Check sheet for the modelled part. Datum: model origin and axes. Units: mm. Face numbers are marked on the shaded views. A direction names the side the tool comes from. Coordinates: 2 decimals unless noted, no trailing zeros. Loops run counter-clockwise (first coordinate to the right, second up) from the corner with the lowest first, then second, coordinate; pieces in that order, holes last. Notation, with made-up numbers: M -38,44.5 L -29,44.5 A8 cw -29,52.5 Z; hole C 76.25,53 d6. An arc over 180 degrees is marked long. Return JSON: item names as keys, results as strings.
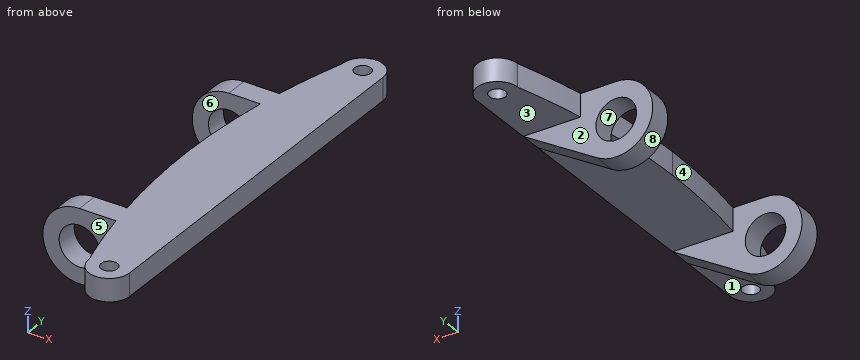
from build123d import *

# Parameters (mm, degrees)
CROQUIS3_R              = 1
SALIENTE_EXTRUIR1_DEPTH = 2.8
SALIENTE_EXTRUIR2_START = 12.5
CROQUIS4_R              = 2.5
SALIENTE_EXTRUIR2_DEPTH = 2.8
SALIENTE_EXTRUIR3_START = -15.3
CROQUIS4_2_R            = 2.5
SALIENTE_EXTRUIR3_DEPTH = 2.8


with BuildPart() as part:
    # Croquis3 → Saliente-Extruir1 (new body)
    with BuildSketch(Plane.XY):
        with BuildLine():
            Line((4.846627727, 23.897818016), (4.846627727, -23.274751548))
            ThreePointArc((4.846627727, -23.274751548), (2.346627727, -25.774751548), (-0.153372273, -23.274751548))
            ThreePointArc((-0.153372273, -23.274751548), (-2.736363907, -11.605217887), (-3.653372273, 0.311533234))
            ThreePointArc((-3.653372273, 0.311533234), (-2.736363907, 12.228284355), (-0.153372273, 23.897818016))
            ThreePointArc((-0.153372273, 23.897818016), (2.346627727, 26.397818016), (4.846627727, 23.897818016))
        make_face()
        with Locations((2.346627727, 23.897818016)):
            Circle(CROQUIS3_R, mode=Mode.SUBTRACT)
        with Locations(Location((2.346627727, -23.274751548, 0), (0, 0, 180))):
            Circle(CROQUIS3_R, mode=Mode.SUBTRACT)
    extrude(amount=SALIENTE_EXTRUIR1_DEPTH)

    # Croquis4 → Saliente-Extruir2 (add)
    with BuildSketch(Plane(origin=(0, 0, 0), x_dir=(1, 0, 0), z_dir=(0, 1, 0)).offset(SALIENTE_EXTRUIR2_START)):
        with BuildLine():
            Line((4.846627727, 0), (-4.267297244, 5.544479263))
            ThreePointArc((-4.267297244, 5.544479263), (-10.939117757, 2.914463527), (-6.606095909, -2.8))
            Line((-6.606095909, -2.8), (-3.653372273, -2.8))
            Line((-3.653372273, -2.8), (4.846627727, -2.8))
            Line((4.846627727, -2.8), (4.846627727, 0))
        make_face()
        with Locations(Location((-6.606095909, 1.7, 0), (0, 0, 270))):
            Circle(CROQUIS4_R, mode=Mode.SUBTRACT)
    extrude(amount=SALIENTE_EXTRUIR2_DEPTH)

    # Croquis4_2 → Saliente-Extruir3 (add)
    with BuildSketch(Plane(origin=(0, 0, 0), x_dir=(1, 0, 0), z_dir=(0, 1, 0)).offset(SALIENTE_EXTRUIR3_START)):
        with BuildLine():
            Line((4.846627727, 0), (-4.267297244, 5.544479263))
            ThreePointArc((-4.267297244, 5.544479263), (-10.939117757, 2.914463527), (-6.606095909, -2.8))
            Line((-6.606095909, -2.8), (-3.653372273, -2.8))
            Line((-3.653372273, -2.8), (4.846627727, -2.8))
            Line((4.846627727, -2.8), (4.846627727, 0))
        make_face()
        with Locations(Location((-6.606095909, 1.7, 0), (0, 0, 270))):
            Circle(CROQUIS4_2_R, mode=Mode.SUBTRACT)
    extrude(amount=SALIENTE_EXTRUIR3_DEPTH)


solid = part.part
1) Go/stop test with flat-tipped pins: pin 1 Ø1.8 at (x, y) = (2.35, 23.9) entering from +Z; pin 2 Ø8 at (x, y) = (-6, -3) entering from -Z; pin 3 Ø5 at (x, z) = (1.5, -3) entering from +Y. Record where each tip stops, or that it passes through.
Answers:
{"pin 1": "through", "pin 2": "z = 0", "pin 3": "y = 15.3"}
2) Section check A-A on y = 13. Record the cut outline in (x, z).
Answers:
{"outline": "M -6.61,2.8 A4.5 ccw long -4.27,-5.54 L 4.85,0 L 4.85,2.8 Z; hole C -6.61,-1.7 d5"}
3) Draft check along Z on the marked faces 6, 7 and 8. Enter one of: +Z half, -Z half, draft (parallel to the pull), parting line (faces both ways), or undercut.
Answers:
{"face 6": "draft", "face 7": "undercut", "face 8": "parting line"}
4) Scan lines: line 1 along Y through (x, z) = (-9.5, -4.75); line 2 along Z through (x, y) = (1.75, -17); line 3 along Z through (x, y) = (-7, 14.5). Record each from-to range of solid material in increasing order. Write a range as [from, to].
Answers:
{"line 1": "[-15.3, -12.5], [12.5, 15.3]", "line 2": "[0, 2.8]", "line 3": "[-6.18, -4.17], [0.77, 2.78]"}
5) Set-up check for the marked faces 1, 2, 3, 4 and 5: record each of +Z, -Z, +X, -X, +Y, -Y from which the full face is reachable in a straight line by a thin tool's end or side.
Answers:
{"face 1": "-Z, +X, -X, -Y", "face 2": "-Z, -X, +Y", "face 3": "-Z, +X, -X, +Y", "face 4": "+Z, -Z, -X", "face 5": "-Z, -X, -Y"}
6) Section check D-D on x = -10. Record the cut outline in (y, z).
Answers:
{"outline": "M -15.3,-4.65 L -12.5,-4.65 L -12.5,1.25 L -15.3,1.25 Z; M 12.5,-4.65 L 15.3,-4.65 L 15.3,1.25 L 12.5,1.25 Z"}
7) Section check B-B on z = 1.5. Record the cut outline in (x, y), then the cut area to 3 significant figures.
Answers:
{"outline": "M -9.77,-15.3 L -2.1,-15.3 A84.82 ccw -0.15,-23.27 A2.5 ccw 4.85,-23.27 L 4.85,23.9 A2.5 ccw -0.15,23.9 A84.82 ccw -2.22,15.3 L -9.77,15.3 L -9.77,12.5 L -2.7,12.5 A84.82 ccw -3.65,0.31 A84.82 ccw -2.6,-12.5 L -9.77,-12.5 Z; hole C 2.35,-23.27 d2; hole C 2.35,23.9 d2", "area": "400 mm²"}
8) Section check C-C on z = -3.5. Record the cut outline in (x, y), then the cut area to 3 significant figures.
Answers:
{"outline": "M -10.73,-15.3 L -8.34,-15.3 L -8.34,-12.5 L -10.73,-12.5 Z; M -10.73,12.5 L -8.34,12.5 L -8.34,15.3 L -10.73,15.3 Z; M -4.87,-15.3 L -0.91,-15.3 L -0.91,-12.5 L -4.87,-12.5 Z; M -4.87,12.5 L -0.91,12.5 L -0.91,15.3 L -4.87,15.3 Z", "area": "35.6 mm²"}
